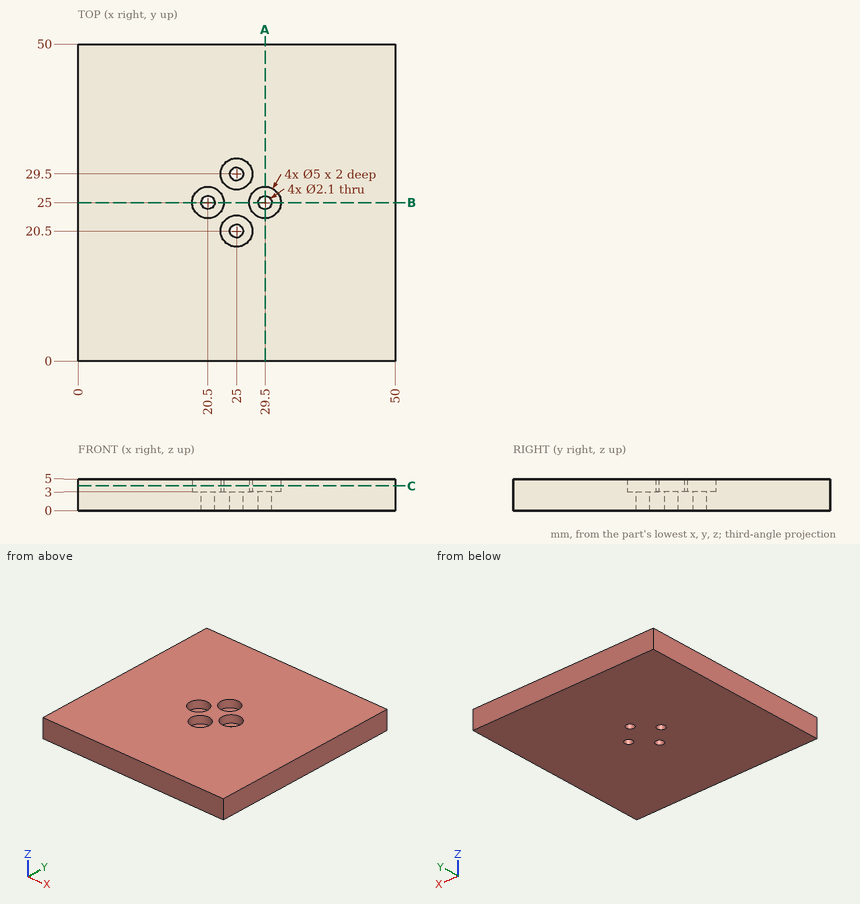
The figure shows three views and two pictorial views of one solid part (mm, origin at its lowest corner). Answer the questions. Coordinates: 2 decimals unless noted, no trailing zeros. Loops run counter-clockwise (first coordinate to the right, second up) from the corner with the lowest first, then second, coordinate; pieces in that order, holes last. Notation, with made-up numbers: M 87,56 L 99,56 A22 ccw 99,78 Z; hole C 76.25,0.25 d7. An arc over 180 degrees is marked long. Use CSV: the item, a comma, the result in double quotes. Start each with the question number.
(1) Given pin 1 Ø2.5 at (x, y) = (20.5, 25) entering from +Z, flat-ended and moving along its own axis, determine where the tip first touches the part or whether it passes through.
(2) Find section C-C, the plane z = 3.9. Give the vertices of the cut face in (x, y), then the cut area to 3 significant figures.
(3) Find section A-A, the plane x = 29.5. Give the vertices of the cut face in (y, z), then the cut area to 3 significant figures.
(4) Consider line 1 (X direction, y = 25, z = 4); line 2 (Y direction, x = 30.5, z = 3.8). Determine where each line is inside the solid, lowest interval first.
(5) Find section B-B, the plane y = 25. Give the vertices of the cut face in (x, z), then the cut area to 3 significant figures.
Recorded:
1,pin 1,"stops at z = 3"
2,outline,"M 0,0 L 50,0 L 50,50 L 0,50 Z; hole C 20.5,25 d5; hole C 25,20.5 d5; hole C 25,29.5 d5; hole C 29.5,25 d5"
2,area,"2,420 mm^2"
3,outline,"M 0,0 L 23.95,0 L 23.95,3 L 22.5,3 L 22.5,5 L 0,5 Z; M 26.05,0 L 50,0 L 50,5 L 27.5,5 L 27.5,3 L 26.05,3 Z"
3,area,"234 mm^2"
4,line 1,"x = 0 to 18, 23 to 27, 32 to 50"
4,line 2,"y = 0 to 22.71, 27.29 to 50"
5,outline,"M 0,0 L 19.45,0 L 19.45,3 L 18,3 L 18,5 L 0,5 Z; M 21.55,0 L 28.45,0 L 28.45,3 L 27,3 L 27,5 L 23,5 L 23,3 L 21.55,3 Z; M 30.55,0 L 50,0 L 50,5 L 32,5 L 32,3 L 30.55,3 Z"
5,area,"217 mm^2"
